CAD build for the part. Positions are in the model's coordinates, mm. A direction names the side the tool comes from. Round coordinates to 2 decimals unless told otherwise and drop trailing zeros. Write each loop counter-clockwise with the first axis right and the second up, starting at its lowest first coordinate (ties: lowest second). Pieces come first, ordered by that corner, then holes. Notation, with made-up numbers: (74.25, 79.5) - (87.25, 79.5) arc R30 ccw to (87.25, 110.5) - close; hole circle Ø2 at (32, 49). An arc over 180 degrees is marked (long way). Use one line per item in the form item = value. Start each with the question number.
Item 1: Tool access for faces 1 (the flat face through (-19, -24, 6)), 2 (the cylindrical face through (18.54, 29.43, 9.4)), 3 (the flat face through (-15.5, -27, 5)), 4 (the flat face through (-21.5, 0, 1)), 5 (the flat face through (0, 0, 2)): list every direction of +Z, -Z, +X, -X, +Y, -Y with a clear straight run to the whole face (end or side of a thin tool).
Item 2: Pull direction Y, two halves, no side cores. Call faces 6 (the cylindrical face through (18.54, -29.43, 9.4)), 7 (the flat face through (15.5, -27, 5)), 8 (the flat face through (-19, 24, 6)): +Y half, -Y half, draft (parallel to the pull), parting line (faces both ways), or undercut.
Item 3: Pin check, flat tips, straight feed: pin 1 (4 mm diameter, centred on x = 14, y = 14, fed in from +Z); pin 2 (3 mm diameter, centred on x = -1, z = 5, fed in from +Y). Stop position of each tip, or through.
Item 4: Band-saw the part on C-C, the plane y = 11.5. List the corners of the cut face in (x, z).
Item 5: Band-saw the part on D-D, the plane x = 13. List the corners of the cut face in (y, z).
Item 6: Band-saw the part on A-A, the plane z = 7. Give the number of separate pieces and of enclosed holes in the cut face, and give its area (3 significant figures).
Item 7: Band-saw the part on B-B, the plane y = -27. List the corners of the cut face in (x, z), and give its area (3 significant figures).
Item 8: Drill centre lines: L1, parallel to Z at x = 18.1, y = 27; L2, parallel to X at y = 24.5, z = 5.25; L3, parallel to Z at x = 10, y = -17.5. Where is each one in solid material? Low to high.
from build123d import *

# Parameters (mm, degrees)
SKETCH_W        = 43
SKETCH_H        = 60
PAD_DEPTH       = 2
SKETCH001_W     = 6
SKETCH001_H     = 6
PAD001_DEPTH    = 8
SKETCH002_R     = 1.5
POCKET_DEPTH    = 6
SKETCH003_R     = 1.5
POCKET001_DEPTH = 6
FILLET_R        = 2
FILLET001_R     = 2
FILLET002_R     = 2
FILLET003_R     = 2


with BuildPart() as part:
    # Sketch → Pad (new body)
    with BuildSketch(Plane.XY):
        Rectangle(SKETCH_W, SKETCH_H)
    extrude(amount=PAD_DEPTH)

    # Sketch001 (on Face6 of Pad) → Pad001 (join)
    with BuildSketch(Plane.XY.offset(2)):
        with Locations((-18.5, 27)):
            Rectangle(SKETCH001_W, SKETCH001_H)
        with Locations((18.5, 27)):
            Rectangle(SKETCH001_W, SKETCH001_H)
        with Locations((-18.5, -27)):
            Rectangle(SKETCH001_W, SKETCH001_H)
        with Locations((18.5, -27)):
            Rectangle(SKETCH001_W, SKETCH001_H)
    extrude(amount=PAD001_DEPTH)

    # Sketch002 (on Face12 of Pad001) → Pocket (cut)
    with BuildSketch(Plane.YZ.offset(21.5)):
        with Locations((-27, 7)):
            Circle(SKETCH002_R)
        with Locations((27, 7)):
            Circle(SKETCH002_R)
    extrude(amount=-POCKET_DEPTH, mode=Mode.SUBTRACT)

    # Sketch003 (on Face10 of Pocket) → Pocket001 (cut)
    with BuildSketch(Plane(origin=(-21.5, 0, 0), x_dir=(0, -1, 0), z_dir=(-1, 0, 0))):
        with Locations((-27, 7)):
            Circle(SKETCH003_R)
        with Locations((27, 7)):
            Circle(SKETCH003_R)
    extrude(amount=-POCKET001_DEPTH, mode=Mode.SUBTRACT)

    # Fillet
    fillet_edges = [part.edges().sort_by_distance(p)[0] for p in [
        (18.5, 30, 10),
    ]]
    fillet(fillet_edges, radius=FILLET_R)

    # Fillet001
    fillet001_edges = [part.edges().sort_by_distance(p)[0] for p in [
        (-18.5, 30, 10),
    ]]
    fillet(fillet001_edges, radius=FILLET001_R)

    # Fillet002
    fillet002_edges = [part.edges().sort_by_distance(p)[0] for p in [
        (-18.5, -30, 10),
    ]]
    fillet(fillet002_edges, radius=FILLET002_R)

    # Fillet003
    fillet003_edges = [part.edges().sort_by_distance(p)[0] for p in [
        (18.5, -30, 10),
    ]]
    fillet(fillet003_edges, radius=FILLET003_R)


solid = part.part
Determined:
q1.face_1 = +Z, +X, -X
q1.face_2 = +Z, +X, -X, +Y
q1.face_3 = +Z, +Y, -Y
q1.face_4 = +Z, -Z, -X, +Y, -Y
q1.face_5 = +Z
q2.face_6 = -Y half
q2.face_7 = draft
q2.face_8 = undercut
q3.pin_1 = 2
q3.pin_2 = through
q4.outline = (-21.5, 0) - (21.5, 0) - (21.5, 2) - (-21.5, 2) - close
q5.outline = (-30, 0) - (30, 0) - (30, 2) - (-30, 2) - close
q6.separate_pieces = 8
q6.enclosed_holes = 0
q6.area = 72.0 mm²
q7.outline = (-21.5, 0) - (21.5, 0) - (21.5, 5.5) - (15.5, 5.5) - (15.5, 2) - (-15.5, 2) - (-15.5, 5.5) - (-21.5, 5.5) - close; (-21.5, 8.5) - (-15.5, 8.5) - (-15.5, 10) - (-21.5, 10) - close; (15.5, 8.5) - (21.5, 8.5) - (21.5, 10) - (15.5, 10) - close
q7.area = 146 mm²
q8.L1 = 0 to 5.5, 8.5 to 10
q8.L2 = -21.5 to -15.5, 15.5 to 21.5
q8.L3 = 0 to 2
